Check sheet for the modelled part. Datum: model origin and axes. Units: mm. Face numbers are marked on the shaded views. Round coordinates to 2 decimals unless told otherwise and drop trailing zeros. Loops run counter-clockwise (first coordinate to the right, second up) from the corner with the lowest first, then second, coordinate; pieces in that order, holes last. Notation, with made-up numbers: (-3, 8) -> (56, 8) arc R35 ccw to (56, 43) -> close; hole circle Ø4 at (38, 0). An arc over 180 degrees is marked (long way). One line per question, with ' | ' between items.
Autodesk Inventor part; units mm, degrees
ref_plane "YZ Plane" through (0, 0, 0) normal (1, 0, 0) x (0, 1, 0)
ref_plane "XZ Plane" through (0, 0, 0) normal (0, 1, 0) x (-1, 0, 0)
ref_plane "XY Plane" through (0, 0, 0) normal (0, 0, 1) x (1, 0, 0)
sketch "Sketch1" plane through (0, 0, 0) normal (1, 0, 0) x (0, 1, 0)
  line L0 (-22.225, 0.762) -> (22.225, 0.762)
  line L1 (22.225, -0.762) -> (-22.225, -0.762)
  line L2 (-22.225, -0.762) -> (-22.225, 0.762)
  line L3 (-22.225, 0.762) -> (22.225, -0.762) construction
  line L4 (22.225, 0.762) -> (-22.225, -0.762) construction
  line L5 (22.225, 0.762) -> (51.435, 64.262)
  line L6 (51.435, 64.262) -> (51.435, 62.738)
  line L7 (51.435, 62.738) -> (22.225, -0.762)
  line L8 (0, -0.762) -> (0, -111.887)
  line L9 (0, -111.887) -> (16.3991, -111.887)
  point P0 (0, 0)
  dimension "d1" = 44.45
  dimension "d2" = 63.5
  dimension "d5" = 1.524
  dimension "d6" = 111.125
  dimension "d8" = 29.21
  dimension "d9" = 1.524
revolve "Revolution1" add sketch "Sketch1" angle 360 about axis through (0, 0, -111.887) along (0, 1, 0)
sketch "Sketch2" plane through (0, 51.435, -111.887) normal (0, 1, 0) x (1, 0, 0)
  circle A0 centre (0, 0) radius 111.125
  circle A1 centre (0, 0) radius 176.149
  line L0 (26.2346, -174.1844) -> (-24.5654, -174.1844) construction
  arc A2 (26.2346, -174.1844) -> (97.3464, -146.8065) centre (0, 0) ccw
  line L1 (0, 0) -> (26.2346, -174.1844) construction
  line L2 (0, 0) -> (97.3464, -146.8065) construction
  arc A3 (16.5503, -109.8856) -> (61.4117, -92.6141) centre (0, 0) ccw
  line L3 (16.5503, -109.8856) -> (26.2346, -174.1844)
  line L4 (97.3464, -146.8065) -> (61.4117, -92.6141)
  dimension "d19" = 50.8
  dimension "d20" = 76.2
extrude "Extrusion2" cut sketch "Sketch2" against normal blind 25.4 contours A0 L4 A1 L3 picked at (28.0302, -151.7692)
pattern_circular "Circular Pattern2" count 8 over 360 about axis through (0, 36.83, -111.887) along (0, 1, 0) of "Extrusion2"
properties part number "rubber_sleeve" material "Rubber"
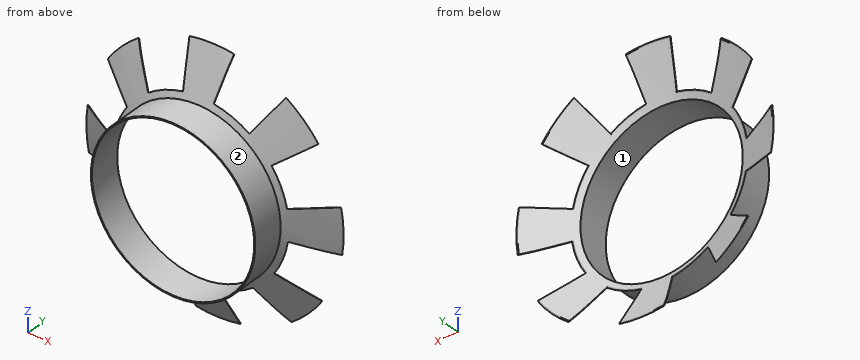
(1) Sectioned sample at C-C, the plane y = -10.5. Record the cut outline in (x, z) (3 decimals).
Answer:
outline: circle Ø225.298 at (0, -111.887); hole circle Ø222.25 at (0, -111.887)
(2) Mould release check, pull along X, two halves, no side actions. Record for the marked faces 1 and 2: +X half, -X half, draft (parallel to the pull), parting line (faces both ways), or undercut.
Answer:
face 1: undercut | face 2: parting line
(3) Scan lines: probe 1 along X at (y, z) = (22.5, -161); probe 2 along X at (y, z) = (-2, -60); probe 3 along Z at (x, y) = (29, 20). Record each from-to range of solid material in increasing order.
Answer:
probe 1: x = -102.04 to -100.35, 100.35 to 102.04 | probe 2: x = -99.99 to -98.27, 98.27 to 99.99 | probe 3: z = -220.74 to -219.16, -4.61 to -3.03
(4) Go/stop test with flat-tipped pins: pin 1 (22 mm diameter, centred on x = -30.5, z = -225, fed in from +Y) (3 decimals); pin 2 (6 mm diameter, centred on y = 31.5, z = -80.5, fed in from -X); pin 3 (12 mm diameter, centred on x = -61, y = -7.5, fed in from +Z); pin 4 (2 mm diameter, centred on y = 10.5, z = -160, fed in from -X). Record where each tip stops, or that it passes through.
Answer:
pin 1: stops at y = 26.035 | pin 2: passes through | pin 3: stops at z = -13.58 | pin 4: stops at x = -102.32
(5) Sectioned sample at A-A, the plane x = 0. Record the cut outline in (y, z) (3 decimals).
Answer:
outline: (-22.225, -224.536) -> (22.225, -224.536) -> (51.435, -288.036) -> (51.435, -286.512) -> (22.225, -223.012) -> (-22.225, -223.012) -> close; (-22.225, -0.762) -> (22.225, -0.762) -> (51.435, 62.738) -> (51.435, 64.262) -> (22.225, 0.762) -> (-22.225, 0.762) -> close
